Geometry: see drawing. Coordinates: mm, zero at the bounding-box minimum. Round coordinates to 2 decimals unless told otherwise and drop trailing zeros. Loops run counter-clockwise (first coordinate to the right, second up) from the corner with the lowest first, then second, coordinate; pieces in that order, holes last. Notation, with made-up numbers: (16.25, 14) - (48.25, 14) arc R19 ccw to (48.25, 37) - close; hole circle Ø9 at (25.25, -31). An arc over 180 degrees is marked (long way). Answer in a Markdown table with one row per item. Add a question column.
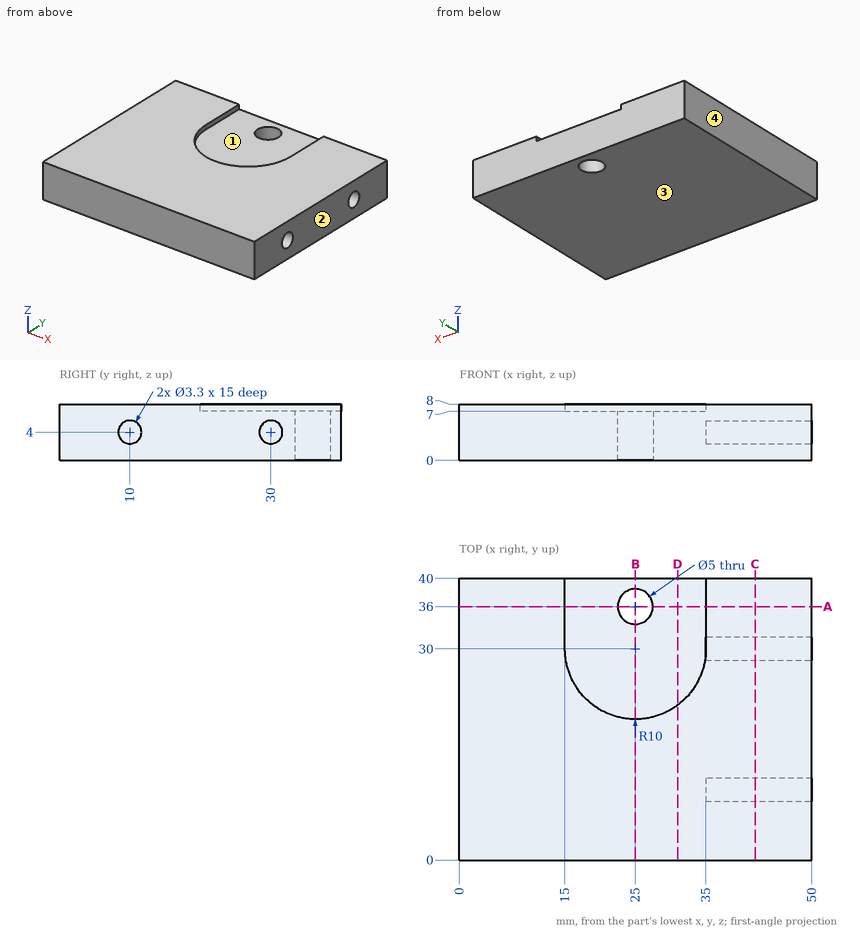
1) Section D-D, the plane x = 31. Return the cut outline in (y, z).
2) Section A-A, the plane y = 36. Return the cut outline in (x, z), and give its area (3 significant figures).
3) Pull-direction query (X, two-part tool) for the marked faces 1, 2, 3 and 4; classes: pulls with the +X half, pulls with the -X half, needs draft (parallel to the pull), parting line crosses it, or undercut.
4) Material intervals for line 1 along Y through (x, z) = (25, 3.25); line 2 along Z through (x, y) = (38.5, 10); line 3 along Y through (x, z) = (44, 3.5), sorted ascending. Write a range as from..to.
5) Contact query for flat-ended pins moving along their axis: pin 1 Ø6 at (x, y) = (20, 25.5) entering from +Z; pin 2 Ø1 at (y, z) = (9.5, 4) entering from +X. Output: stop coordinate, or through.
6) Section C-C, the plane x = 42. Return the cut outline in (y, z), and give its area (3 significant figures).
7) Section B-B, the plane x = 25. Return the cut outline in (y, z), and give its area (3 significant figures).
Evaluation:
| question | item | result |
|---|---|---|
| 1 | outline | (0, 0) - (40, 0) - (40, 7) - (22, 7) - (22, 8) - (0, 8) - close |
| 2 | outline | (0, 0) - (22.5, 0) - (22.5, 7) - (15, 7) - (15, 8) - (0, 8) - close; (27.5, 0) - (50, 0) - (50, 8) - (35, 8) - (35, 7) - (27.5, 7) - close |
| 2 | area | 345 mm² |
| 3 | face 1 | undercut |
| 3 | face 2 | pulls with the +X half |
| 3 | face 3 | needs draft |
| 3 | face 4 | pulls with the -X half |
| 4 | line 1 | y = 0..33.5, 38.5..40 |
| 4 | line 2 | z = 0..2.35, 5.65..8 |
| 4 | line 3 | y = 0..8.43, 11.57..28.43, 31.57..40 |
| 5 | pin 1 | stops at z = 7 |
| 5 | pin 2 | stops at x = 35 |
| 6 | outline | (0, 0) - (40, 0) - (40, 8) - (0, 8) - close; hole circle Ø3.3 at (10, 4); hole circle Ø3.3 at (30, 4) |
| 6 | area | 303 mm² |
| 7 | outline | (0, 0) - (33.5, 0) - (33.5, 7) - (20, 7) - (20, 8) - (0, 8) - close; (38.5, 0) - (40, 0) - (40, 7) - (38.5, 7) - close |
| 7 | area | 265 mm² |
